Study the drawing (mm; zero at the part's minimum x, y, z) and answer. Coordinates: 2 decimals unless noted, no trailing zeros. Order: outer loops, then holes, each group sorted by start corner. A loop starts at its lowest first (then second) coordinate and runs counter-clockwise, first axis right, second up. Notation, with made-up numbers: M -14,-1 L -8,-1 A36 cw -8,34 Z; hole C 27,46.25 d10. An arc over 180 degrees is marked long. One line per item, written item: value. Start each with the question number.
Q1. The part is cut by section C-C on z = 3.05. Give the number of separate pieces and of enclosed holes in the cut face, then the cut area to 3 significant figures.
Q2. The part is cut by section A-A on x = 80.01. Give the vertices of the cut face in (y, z), then the cut area to 3 significant figures.
Q3. Straight lines are drawn through the part: line 1 along X through (y, z) = (29.21, 3) (1 decimal); line 2 along X through (y, z) = (19.05, 3.65) (1 decimal); line 3 along X through (y, z) = (8.89, 1.05) (1 decimal). For each, find the intervals that lie inside material, in ascending order. Write a range as [from, to].
Q4. The part is cut by section D-D on x = 201.93. Give the vertices of the cut face in (y, z) (1 decimal).
Q5. The part is cut by section B-B on y = 19.05. Give the vertices of the cut face in (x, z) (1 decimal).
Q6. This flat-tipped pin is pushed along its axis until it touches: pin 1 Ø5 at (x, y) = (214.63, 29.21) entering from +Z. Where does it stop, or does it pass through?
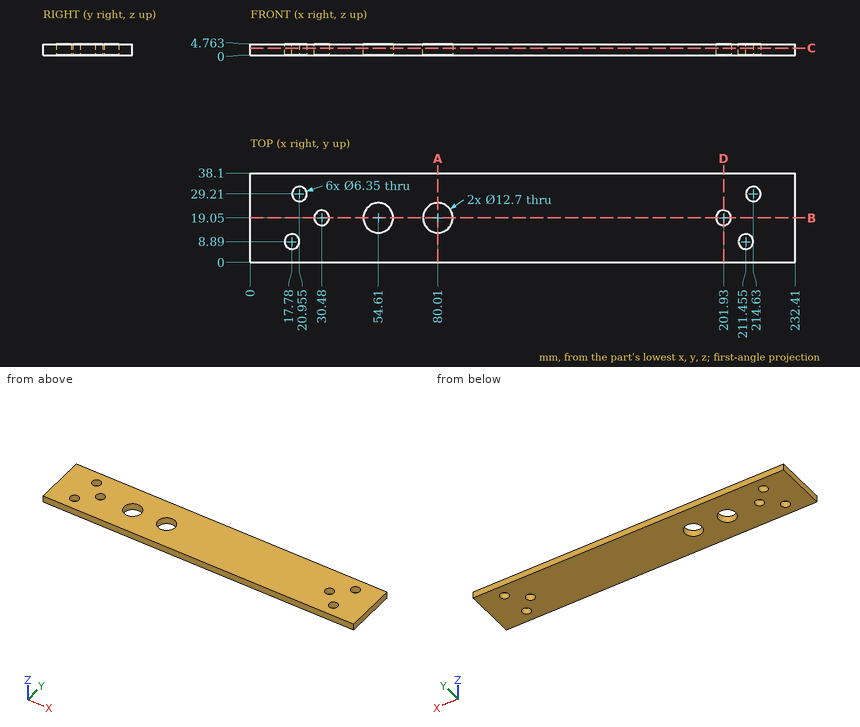
Output:
1. separate pieces: 1
1. enclosed holes: 8
1. area: 8,410 mm^2
2. outline: M 0,0 L 12.7,0 L 12.7,4.76 L 0,4.76 Z; M 25.4,0 L 38.1,0 L 38.1,4.76 L 25.4,4.76 Z
2. area: 121 mm^2
3. line 1: x = [0, 17.8], [24.1, 211.5], [217.8, 232.4]
3. line 2: x = [0, 27.3], [33.7, 48.3], [61, 73.7], [86.4, 198.8], [205.1, 232.4]
3. line 3: x = [0, 14.6], [21, 208.3], [214.6, 232.4]
4. outline: M 0,0 L 15.9,0 L 15.9,4.8 L 0,4.8 Z; M 22.2,0 L 38.1,0 L 38.1,4.8 L 22.2,4.8 Z
5. outline: M 0,0 L 27.3,0 L 27.3,4.8 L 0,4.8 Z; M 33.7,0 L 48.3,0 L 48.3,4.8 L 33.7,4.8 Z; M 61,0 L 73.7,0 L 73.7,4.8 L 61,4.8 Z; M 86.4,0 L 198.8,0 L 198.8,4.8 L 86.4,4.8 Z; M 205.1,0 L 232.4,0 L 232.4,4.8 L 205.1,4.8 Z
6. pin 1: passes through
